Could you check a few things on this model? Use its own coordinates, in mm. Coordinates: 2 decimals unless noted, no trailing zeros. Loops run counter-clockwise (first coordinate to the right, second up) from the corner with the lowest first, then second, coordinate; pieces in that order, holes last. Notation, with made-up numbers: (35, 71.25) - (53, 71.25) arc R10 ccw to (53, 79.25) - close; hole circle Ø5 at (24.5, -32.5). An arc over 180 degrees is marked (long way). Use CSV: the item, a comma, the result in double quotes.
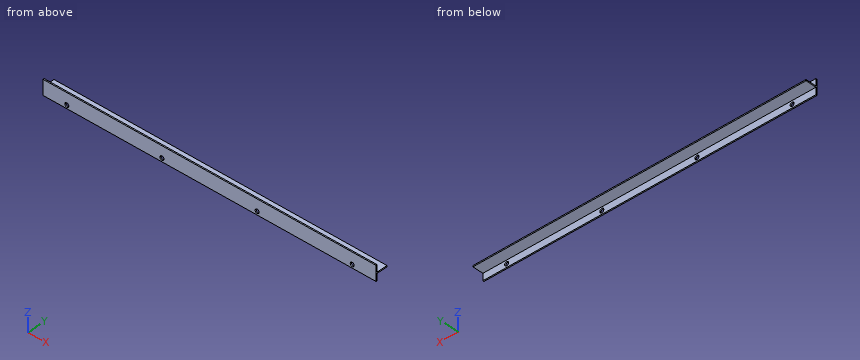
from build123d import *

# Parameters (mm, degrees)
BOSS_EXTRUDE1_DEPTH = 355.6
CUT_EXTRUDE1_REACH  = 3.27
SKETCH2_R           = 2.15265


with BuildPart() as part:
    # Sketch1 → Boss-Extrude1 (new body)
    with BuildSketch(Plane(origin=(0, 0, 0), x_dir=(0, 0, -1), z_dir=(1, 0, 0))):
        Polygon((0.635, 0), (7.9375, 0), (7.9375, -1.27), (-7.9375, -1.27), (-7.9375, 0), (-0.635, 0), (-0.635, 11.43), (0.635, 11.43), align=None)
    extrude(amount=BOSS_EXTRUDE1_DEPTH)

    # Sketch2 → Cut-Extrude1 (cut, up to next)
    with BuildSketch(Plane(origin=(0, 0, 0), x_dir=(1, 0, 0), z_dir=(0, 1, 0)), mode=Mode.PRIVATE) as cut_extrude1_sk1:
        with Locations((25.4, 4.28625)):
            Circle(SKETCH2_R)
    cut_extrude1_tool1 = extrude(cut_extrude1_sk1.sketch, amount=-CUT_EXTRUDE1_REACH, mode=Mode.PRIVATE) & part.part
    add(cut_extrude1_tool1.solids().sort_by_distance((25.4, 0, -4.28625))[0], mode=Mode.SUBTRACT)
    # Sketch2 → Cut-Extrude1 (cut, up to next)
    with BuildSketch(Plane(origin=(0, 0, 0), x_dir=(1, 0, 0), z_dir=(0, 1, 0)), mode=Mode.PRIVATE) as cut_extrude1_sk2:
        with Locations((127, 4.28625)):
            Circle(SKETCH2_R)
    cut_extrude1_tool2 = extrude(cut_extrude1_sk2.sketch, amount=-CUT_EXTRUDE1_REACH, mode=Mode.PRIVATE) & part.part
    add(cut_extrude1_tool2.solids().sort_by_distance((127, 0, -4.28625))[0], mode=Mode.SUBTRACT)
    # Sketch2 → Cut-Extrude1 (cut, up to next)
    with BuildSketch(Plane(origin=(0, 0, 0), x_dir=(1, 0, 0), z_dir=(0, 1, 0)), mode=Mode.PRIVATE) as cut_extrude1_sk3:
        with Locations((228.6, 4.28625)):
            Circle(SKETCH2_R)
    cut_extrude1_tool3 = extrude(cut_extrude1_sk3.sketch, amount=-CUT_EXTRUDE1_REACH, mode=Mode.PRIVATE) & part.part
    add(cut_extrude1_tool3.solids().sort_by_distance((228.6, 0, -4.28625))[0], mode=Mode.SUBTRACT)
    # Sketch2 → Cut-Extrude1 (cut, up to next)
    with BuildSketch(Plane(origin=(0, 0, 0), x_dir=(1, 0, 0), z_dir=(0, 1, 0)), mode=Mode.PRIVATE) as cut_extrude1_sk4:
        with Locations((330.2, 4.28625)):
            Circle(SKETCH2_R)
    cut_extrude1_tool4 = extrude(cut_extrude1_sk4.sketch, amount=-CUT_EXTRUDE1_REACH, mode=Mode.PRIVATE) & part.part
    add(cut_extrude1_tool4.solids().sort_by_distance((330.2, 0, -4.28625))[0], mode=Mode.SUBTRACT)


solid = part.part
(1) Please list where these lines run through material, in increasing order: line 1 (Z direction, x = 127, y = -0.95); line 2 (Y direction, x = 112, z = 3); line 3 (Z direction, x = 72, y = 1.5) (3 decimals).
Computed:
line 1,"z = -7.94 to -6.44, -2.13 to 7.94"
line 2,"y = -1.27 to 0"
line 3,"z = -0.635 to 0.635"
(2) Suppose I cut it at A-A (x = 274). Write out the boundary of the cut face in (y, z) (1 decimal), plus the area to 3 significant figures.
Computed:
outline,"(-1.3, -7.9) - (0, -7.9) - (0, -0.6) - (11.4, -0.6) - (11.4, 0.6) - (0, 0.6) - (0, 7.9) - (-1.3, 7.9) - close"
area,"34.7 mm²"
(3) Will these pins go through, and if not, where does the flat tip stop? pin 1 (4 mm diameter, centred on x = 25.4, z = -4.29, fed in from +Y); pin 2 (6 mm diameter, centred on x = 198.5, z = -6, fed in from +Y); pin 3 (3.5 mm diameter, centred on x = 156.5, y = 5, fed in from -Z) (3 decimals).
Computed:
pin 1,"passes through"
pin 2,"stops at y = 0"
pin 3,"stops at z = -0.635"
(4) Suppose I cut it at B-B (y = 7.5). Write out the boundary of the cut face in (x, z) (3 decimals), plus the area to 3 significant figures.
Computed:
outline,"(0, -0.635) - (355.6, -0.635) - (355.6, 0.635) - (0, 0.635) - close"
area,"452 mm²"
